Part model, mm, in its own coordinate system. Face numbers are marked on the shaded views. Coordinates: 2 decimals unless noted, no trailing zeros. Loops run counter-clockwise (first coordinate to the right, second up) from the corner with the lowest first, then second, coordinate; pieces in that order, holes last. Notation, with made-up numbers: (53.25, 40.25) - (101.25, 40.25) arc R16 cw to (101.25, 49.25) - close; hole circle Ø10 at (86.25, 25). An arc over 180 degrees is marked (long way). Use a Markdown table: item, result. Add a question column.
1. Pull direction X, two halves, no side cores. Call the marked faces 1, 2 and 3: pulls with the +X half, pulls with the -X half, needs draft (parallel to the pull), parting line crosses it, or undercut.
2. Wall check: probe 1 along X at (y, z) = (6.5, 3.5); probe 2 along Z at (x, y) = (5, 5.75) (3 decimals); probe 3 along X at (y, z) = (7.5, 22). Give the ranges that are in metal, low to high. Write a range as [from, to].
3. Band-saw the part on C-C, the plane x = 12.75. Give the cut face in (y, z) (3 decimals).
4. Band-saw the part on D-D, the plane y = 9.75. Give the cut face in (x, z) (3 decimals), plus the area to 3 significant figures.
5. Band-saw the part on A-A, the plane z = 25.5. Give the cut face in (x, y), plus the area to 3 significant figures.
6. Band-saw the part on B-B, the plane y = 6.35. Give the cut face in (x, z) (3 decimals), plus the area to 3 significant figures.
7. Drop flat-ended pins along their axis: pin 1 (3 mm diameter, centred on x = 6.5, y = 5, fed in from +Z) (3 decimals); pin 2 (6 mm diameter, centred on y = 5, z = 16, fed in from -X); pin 3 (1.5 mm diameter, centred on y = 4.5, z = 11, fed in from -X). Give the stop position or say it passes through.
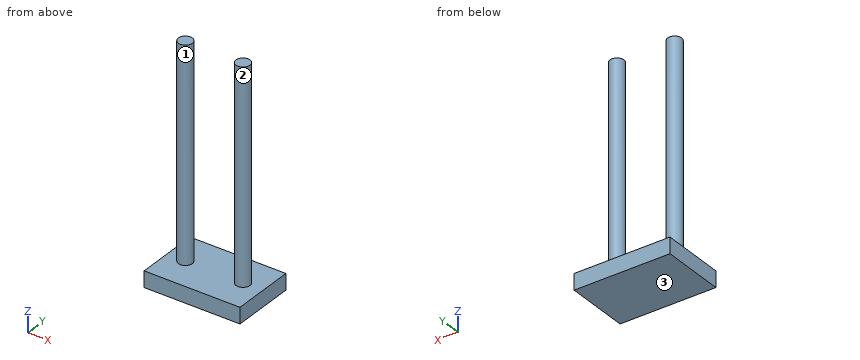
from build123d import *

# Parameters (mm, degrees)
F0_W     = 19.05
F0_H     = 12.7
F1_DEPTH = 3.175
F2_R     = 1.397
F3_DEPTH = 6.35
F4_R     = 1.397
F5_DEPTH = 35.56


with BuildPart() as f1:
    # F0 (on Top) → F1 (new body)
    with BuildSketch(Plane.XY):
        with Locations((9.525, 6.35)):
            Rectangle(F0_W, F0_H)
    extrude(amount=F1_DEPTH)

    # F2 (on face) → F3 (join)
    with BuildSketch(Plane.XY.offset(3.175)):
        with Locations((3.643117, 6.35)):
            Circle(F2_R)
        with BuildLine():
            ThreePointArc((16.495517, 6.35), (15.098517, 7.747), (13.701517, 6.35))
            ThreePointArc((13.701517, 6.35), (15.098517, 4.953), (16.495517, 6.35))
        make_face()
    extrude(amount=F3_DEPTH)

    # F4 (on face) → F5 (join)
    with BuildSketch(Plane.XY.offset(9.525)):
        with Locations((3.643117, 6.35)):
            Circle(F4_R)
        with BuildLine():
            ThreePointArc((16.495517, 6.35), (15.098517, 7.747), (13.701517, 6.35))
            ThreePointArc((13.701517, 6.35), (15.098517, 4.953), (16.495517, 6.35))
        make_face()
    extrude(amount=F5_DEPTH)


solid = f1.part
Geometry check:
| question | item | result |
|---|---|---|
| 1 | face 1 | undercut |
| 1 | face 2 | undercut |
| 1 | face 3 | needs draft |
| 2 | probe 1 | x = [2.25, 5.03], [13.71, 16.49] |
| 2 | probe 2 | z = [0, 3.175] |
| 2 | probe 3 | x = [2.85, 4.44], [14.31, 15.89] |
| 3 | outline | (0, 0) - (12.7, 0) - (12.7, 3.175) - (0, 3.175) - close |
| 4 | outline | (0, 0) - (19.05, 0) - (19.05, 3.175) - (0, 3.175) - close |
| 4 | area | 60.5 mm^2 |
| 5 | outline | circle Ø2.79 at (3.64, 6.35); circle Ø2.79 at (15.1, 6.35) |
| 5 | area | 12.3 mm^2 |
| 6 | outline | (0, 0) - (19.05, 0) - (19.05, 3.175) - (16.496, 3.175) - (16.496, 45.085) - (13.702, 45.085) - (13.702, 3.175) - (5.04, 3.175) - (5.04, 45.085) - (2.246, 45.085) - (2.246, 3.175) - (0, 3.175) - close |
| 6 | area | 295 mm^2 |
| 7 | pin 1 | stops at z = 3.175 |
| 7 | pin 2 | stops at x = 2.25 |
| 7 | pin 3 | stops at x = 2.78 |
